Geometry check sheet. Reference: the model listing, model coordinates, mm. Give positions to 0.01 mm unless a question says otherwise; leave off trailing zeros. Order: outer loops, then holes, each group sorted by start corner. A loop starts at its lowest first (then second) coordinate and runs counter-clockwise, first axis right, second up. Notation, with made-up numbers: M 70.25,45 L 106.25,45 A13 cw 106.25,57 Z; hole C 74.25,-23.75 d3. An arc over 180 degrees is marked long. Put each result on its own line as item: value. Start each with the question number.
Q1. Mould release check, pull along X, two halves, no side actions. Record for faces 1 (the cylindrical face through (-1.55, -5.53, 12.63)), 2 (the cylindrical face through (3.687, -7.089, 12.522)), 3 (the flat face through (0, 0, 25.4)): +X half, -X half, draft (parallel to the pull), parting line (faces both ways), or undercut.
Q2. Material ranges on L1, parallel to Z at x = 0, y = 6.4; L2, parallel to Y at x = 0.25, z = 8.75; L3, parallel to Z at x = 5.25, y = 0, recorded low to high.
Q3. Go/stop test with flat-tipped pins: pin 1 (2 mm diameter, centred on x = 4.5, y = 1, fed in from -Z); pin 2 (2 mm diameter, centred on y = -1.5, z = 4.5, fed in from +X); pin 3 (3 mm diameter, centred on x = -5.5, z = 12, fed in from +Y); pin 4 (3 mm diameter, centred on y = 4, z = 18.5, fed in from -X). Record where each tip stops, or that it passes through.
Q4. Section check B-B on z = 12.7. Record the cut outline in (x, y).
Q5. Section check D-D on x = 2.75. Record the cut outline in (y, z).
Q6. Section check A-A on y = 0. Record the cut outline in (x, z).
Q7. Section check C-C on x = -0.5. Record the cut outline in (y, z), then the cut area to 3 significant figures.
```python
from build123d import *

# Parameters (mm, degrees)
SKETCH1_R               = 7.99
EXTRUDE1_DEPTH          = 25.4
SKETCH2_R               = 3.5
CUT_EXTRUDE2_DEPTH      = 8.99
CUT_EXTRUDE2_DEPTH_BACK = 8.99
SKETCH3_R               = 1.55
CUT_EXTRUDE3_DEPTH      = 8.9900001
CUT_EXTRUDE3_DEPTH_BACK = 8.9900001


with BuildPart() as part:
    # Sketch1 → Extrude1 (new body)
    with BuildSketch(Plane.XY):
        Circle(SKETCH1_R)
    extrude(amount=EXTRUDE1_DEPTH)

    # Sketch2 → Cut-Extrude2 (cut, two sides)
    with BuildSketch(Plane(origin=(0, 0, 0), x_dir=(0, 0, -1), z_dir=(1, 0, 0))) as cut_extrude2_sk:
        with Locations((-12.7, 0)):
            Circle(SKETCH2_R)
    extrude(amount=CUT_EXTRUDE2_DEPTH, mode=Mode.SUBTRACT)
    extrude(cut_extrude2_sk.sketch, amount=-CUT_EXTRUDE2_DEPTH_BACK, mode=Mode.SUBTRACT)

    # Sketch3 → Cut-Extrude3 (cut, two sides)
    with BuildSketch(Plane(origin=(0, 0, 0), x_dir=(1, 0, 0), z_dir=(0, 1, 0))) as cut_extrude3_sk:
        with Locations((0, -12.7)):
            Circle(SKETCH3_R)
    extrude(amount=CUT_EXTRUDE3_DEPTH, mode=Mode.SUBTRACT)
    extrude(cut_extrude3_sk.sketch, amount=-CUT_EXTRUDE3_DEPTH_BACK, mode=Mode.SUBTRACT)


solid = part.part
```
Results found:
1. face 1: undercut
1. face 2: parting line
1. face 3: draft
2. L1: z = 0 to 11.15, 14.25 to 25.4
2. L2: y = -7.99 to 7.99
2. L3: z = 0 to 9.2, 16.2 to 25.4
3. pin 1: stops at z = 0
3. pin 2: stops at x = 7.97
3. pin 3: stops at y = 6.92
3. pin 4: stops at x = -7.59
4. outline: M -7.18,-3.5 A7.99 ccw -1.55,-7.84 L -1.55,-3.5 Z; M -7.18,3.5 L -1.55,3.5 L -1.55,7.84 A7.99 ccw Z; M 1.55,-7.84 A7.99 ccw 7.18,-3.5 L 1.55,-3.5 Z; M 1.55,3.5 L 7.18,3.5 A7.99 ccw 1.55,7.84 Z
5. outline: M -7.5,0 L 7.5,0 L 7.5,25.4 L -7.5,25.4 Z; hole C 0,12.7 d7
6. outline: M -7.99,0 L 7.99,0 L 7.99,9.2 L -7.99,9.2 Z; M -7.99,16.2 L 7.99,16.2 L 7.99,25.4 L -7.99,25.4 Z
7. outline: M -7.97,0 L 7.97,0 L 7.97,11.23 L 3.18,11.23 A3.5 cw -3.18,11.23 L -7.97,11.23 Z; M -7.97,14.17 L -3.18,14.17 A3.5 cw 3.18,14.17 L 7.97,14.17 L 7.97,25.4 L -7.97,25.4 Z
7. area: 340 mm^2
